```python
from build123d import *

# Parameters (mm, degrees)
CROQUIS1_W                                           = 190
CROQUIS1_H                                           = 200
SALIENTE_EXTRUIR1_DEPTH                              = 15
CROQUIS2_R                                           = 4
CORTAR_EXTRUIR1_DEPTH                                = 139.744369255
CROQUIS3_R                                           = 5
CORTAR_EXTRUIR2_DEPTH                                = 139.744369255
CHAFL_N1_SIZE                                        = 5
REFRENTADO_PARA_TORNILLO_TAP_N_CON_CABEZ_D           = 9
REFRENTADO_PARA_TORNILLO_TAP_N_CON_CABEZ_CBORE_D     = 15
REFRENTADO_PARA_TORNILLO_TAP_N_CON_CABEZ_CBORE_DEPTH = 8


with BuildPart() as part:
    # Croquis1 → Saliente-Extruir1 (new body)
    with BuildSketch(Plane.XY):
        Rectangle(CROQUIS1_W, CROQUIS1_H)
    extrude(amount=SALIENTE_EXTRUIR1_DEPTH)

    # Croquis2 → Cortar-Extruir1 (cut, through all)
    with BuildSketch(Plane.XY.offset(15)):
        with Locations((-40, 80)):
            Circle(CROQUIS2_R)
        with Locations((40, 80)):
            Circle(CROQUIS2_R)
        with Locations((40, -80)):
            Circle(CROQUIS2_R)
        with Locations((-40, -80)):
            Circle(CROQUIS2_R)
    extrude(amount=-CORTAR_EXTRUIR1_DEPTH, mode=Mode.SUBTRACT)

    # Croquis3 → Cortar-Extruir2 (cut, through all)
    with BuildSketch(Plane.XY.offset(15)):
        with Locations((-80, 80)):
            Circle(CROQUIS3_R)
        with Locations((80, 80)):
            Circle(CROQUIS3_R)
        with Locations((80, -80)):
            Circle(CROQUIS3_R)
        with Locations((-80, -80)):
            Circle(CROQUIS3_R)
    extrude(amount=-CORTAR_EXTRUIR2_DEPTH, mode=Mode.SUBTRACT)

    # Chaflán1
    chafl_n1_edges = [part.edges().sort_by_distance(p)[0] for p in [
        (95, -100, 7.5),
        (-95, -100, 7.5),
        (-95, 100, 7.5),
        (95, 100, 7.5),
    ]]
    chamfer(chafl_n1_edges, length=CHAFL_N1_SIZE)

    # Refrentado para tornillo tapón con cabeza de clavija de M81 (through all)
    with Locations(Plane.XY.offset(15)):
        with Locations((40, 80), (-40, 80), (-40, -80), (40, -80)):
            CounterBoreHole(REFRENTADO_PARA_TORNILLO_TAP_N_CON_CABEZ_D / 2, REFRENTADO_PARA_TORNILLO_TAP_N_CON_CABEZ_CBORE_D / 2, REFRENTADO_PARA_TORNILLO_TAP_N_CON_CABEZ_CBORE_DEPTH)


solid = part.part
```
Geometry check sheet. Reference: the model listing, model coordinates, mm. A direction names the side the tool comes from. Coordinates: 2 decimals unless noted, no trailing zeros. Order: outer loops, then holes, each group sorted by start corner. A loop starts at its lowest first (then second) coordinate and runs counter-clockwise, first axis right, second up. Notation, with made-up numbers: M 24,29.5 L 77,29.5 A25 cw 77,68.5 Z; hole C 7,83.5 d2. An arc over 180 degrees is marked long. One line per question, with ' | ' between items. Start each with the question number.
Item 1: Cross-section at B-B on x = -80. Enter the section's corners in (y, z).
Item 2: Draft check along X on faces 1 (the cylindrical face through (38.37, 72.68, 11.06)), 2 (the flat face through (-1, 100, 7)), 3 (the flat face through (-95, -1, 7)). Enter one of: pulls with the +X half, pulls with the -X half, needs draft (parallel to the pull), parting line crosses it, or undercut.
Item 3: Cross-section at C-C on z = 2.25. State how many separate pieces and enclosed holes the cut face has, then the cut area to 3 significant figures.
Item 4: Set-up check for faces 4 (the cylindrical face through (84.619, 78.085, 7.605)), 5 (the flat face through (-35, 80, 7)): record each of +Z, -Z, +X, -X, +Y, -Y from which the full face is reachable in a straight line by a thin tool's end or side.
Item 5: Cross-section at D-D on x = -40. Enter the section's corners in (y, z), then the cut area to 3 significant figures.
Item 6: Gauge pin test, flat ends, axial feed: pin 1 (7.5 mm diameter, centred on x = 37.5, y = 79, fed in from +Z); pin 2 (3 mm diameter, centred on x = 3.5, y = -8.5, fed in from -Z). Record the tip position at first contact, or that the pin passes through.
Item 7: Cross-section at A-A on y = -80. Enter the section's corners in (x, z), then the cut area to 3 significant figures.
Item 8: Material ranges on L1, parallel to Y at x = -80, z = 9.5; L2, parallel to Y at x = 40, z = 12.25; L3, parallel to X at y = 80.5, z = 7.75, recorded low to high. Write a range as [from, to].
Findings:
1) outline: M -100,0 L -85,0 L -85,15 L -100,15 Z; M -75,0 L 75,0 L 75,15 L -75,15 Z; M 85,0 L 100,0 L 100,15 L 85,15 Z
2) face 1: undercut | face 2: needs draft | face 3: pulls with the -X half
3) separate pieces: 1 | enclosed holes: 8 | area: 37,400 mm²
4) face 4: +Z, -Z | face 5: +Z
5) outline: M -100,0 L -84.5,0 L -84.5,7 L -87.5,7 L -87.5,15 L -100,15 Z; M -75.5,0 L 75.5,0 L 75.5,7 L 72.5,7 L 72.5,15 L -72.5,15 L -72.5,7 L -75.5,7 Z; M 84.5,0 L 100,0 L 100,15 L 87.5,15 L 87.5,7 L 84.5,7 Z | area: 2,630 mm²
6) pin 1: stops at z = 7 | pin 2: stops at z = 0
7) outline: M -95,0 L -85,0 L -85,15 L -95,15 Z; M -75,0 L -44.5,0 L -44.5,7 L -47.5,7 L -47.5,15 L -75,15 Z; M -35.5,0 L 35.5,0 L 35.5,7 L 32.5,7 L 32.5,15 L -32.5,15 L -32.5,7 L -35.5,7 Z; M 44.5,0 L 75,0 L 75,15 L 47.5,15 L 47.5,7 L 44.5,7 Z; M 85,0 L 95,0 L 95,15 L 85,15 Z | area: 2,180 mm²
8) L1: y = [-100, -85], [-75, 75], [85, 100] | L2: y = [-100, -87.5], [-72.5, 72.5], [87.5, 100] | L3: x = [-95, -84.97], [-75.03, -47.48], [-32.52, 32.52], [47.48, 75.03], [84.97, 95]
